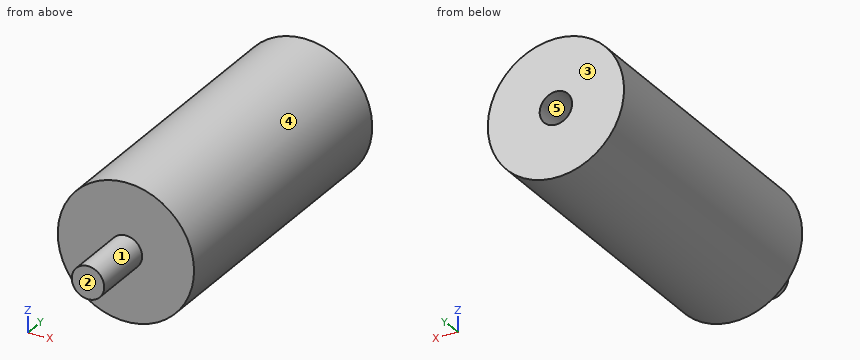
```python
from build123d import *

# Parameters (mm, degrees)
SKETCH1_R           = 10.5
BOSS_EXTRUDE1_DEPTH = 47
SKETCH2_R           = 2.5
CUT_EXTRUDE1_DEPTH  = 10
SKETCH3_R           = 2.5
BOSS_EXTRUDE2_DEPTH = 10


with BuildPart() as part:
    # Sketch1 → Boss-Extrude1 (new body)
    with BuildSketch(Plane(origin=(0, 0, 0), x_dir=(1, 0, 0), z_dir=(0, 1, 0))):
        with Locations(Location((0, 0, 0), (0, 0, 270))):
            Circle(SKETCH1_R)
    extrude(amount=BOSS_EXTRUDE1_DEPTH)

    # Sketch2 → Cut-Extrude1 (cut)
    with BuildSketch(Plane(origin=(0, 47, 0), x_dir=(1, 0, 0), z_dir=(0, 1, 0))):
        with Locations(Location((0, 0, 0), (0, 0, 270))):
            Circle(SKETCH2_R)
    extrude(amount=-CUT_EXTRUDE1_DEPTH, mode=Mode.SUBTRACT)

    # Sketch3 → Boss-Extrude2 (add)
    with BuildSketch(Plane.XZ):
        with Locations(Location((0, 0, 0), (0, 0, 90))):
            Circle(SKETCH3_R)
    extrude(amount=BOSS_EXTRUDE2_DEPTH)


solid = part.part
```
CAD build for the part. Positions are in the model's coordinates, mm. Face numbers are marked on the shaded views. A direction names the side the tool comes from. Give positions to 0.01 mm unless a question says otherwise; leave off trailing zeros. Loops run counter-clockwise (first coordinate to the right, second up) from the corner with the lowest first, then second, coordinate; pieces in that order, holes last. Notation, with made-up numbers: M 27,7 L 78,7 A25 cw 78,25 Z; hole C 66.25,34.25 d11. An arc over 180 degrees is marked long. Use one line per item in the form item = value.
Item 1: Slice it at C-C (y = 43.5). List the corners of the cut face in (x, z).
Determined:
outline = C 0,0 d21; hole C 0,0 d5
Item 2: Which spindle directions (+Z, -Z, +X, -X, +Y, -Y) get a long thin tool onto all of the face, cutting with end or side? Do the marked faces 1 and 2. Say none if no direction does.
Determined:
face_1 = -Y
face_2 = +Z, -Z, +X, -X, -Y
Item 3: Slice it at A-A (x = 0). List the corners of the cut face in (y, z), plus the area to 3 significant figures.
Determined:
outline = M -10,-2.5 L 0,-2.5 L 0,-10.5 L 47,-10.5 L 47,-2.5 L 37,-2.5 L 37,2.5 L 47,2.5 L 47,10.5 L 0,10.5 L 0,2.5 L -10,2.5 Z
area = 987 mm2
Item 4: Two-plate mould, pull along X, no slides. Class the marked faces 3, 4 and 5: pulls with the +X half, pulls with the -X half, needs draft (parallel to the pull), parting line crosses it, or undercut.
Determined:
face_3 = needs draft
face_4 = parting line crosses it
face_5 = undercut
Item 5: Slice it at D-D (y = 20.5). List the corners of the cut face in (x, z), plus the area to 3 significant figures.
Determined:
outline = C 0,0 d21
area = 346 mm2
Item 6: Flat gauge pins, fed straight in: pin 1 (5 mm diameter, centred on x = 7.5, z = -6.5, fed in from -Y); pin 2 (4 mm diameter, centred on x = -6, y = 18, fed in from +Z); pin 3 (3 mm diameter, centred on x = 7.5, y = 22.5, fed in from -Z). Where does each tip first touch, or does it go through?
Determined:
pin_1 = 0
pin_2 = 9.71
pin_3 = -8.62
Item 7: Drill centre lines: probe 1 along X at (y, z) = (42.5, 0); probe 2 along Y at (x, z) = (3, -8.25); probe 3 along X at (y, z) = (19, 0.25). Where is each one in solid material? Low to high. Write a range as from..to.
Determined:
probe_1 = -10.5..-2.5, 2.5..10.5
probe_2 = 0..47
probe_3 = -10.5..10.5
Item 8: Slice it at B-B (z = 0). List the corners of the cut face in (x, y).
Determined:
outline = M -10.5,0 L -2.5,0 L -2.5,-10 L 2.5,-10 L 2.5,0 L 10.5,0 L 10.5,47 L 2.5,47 L 2.5,37 L -2.5,37 L -2.5,47 L -10.5,47 Z
